CAD build for the part. Positions are in the model's coordinates, mm. A direction names the side the tool comes from. Give positions to 0.01 mm unless a question says otherwise; leave off trailing zeros. Write each loop counter-clockwise with the first axis right and the second up, starting at its lowest first coordinate (ties: lowest second). Pieces come first, ordered by that corner, then holes. Notation, with made-up numbers: (-12, -10.75) - (7, -10.75) arc R28 cw to (7, 20.25) - close; hole circle Ø8 at (-24, 46). An arc over 180 degrees is marked (long way). Answer as a JSON object with one key per item and string values.
from build123d import *

# Parameters (mm, degrees)
F0_R      = 1.778
F1_DEPTH  = 1.5875
F3_DEPTH  = 31.75
F4_R      = 2.921
F4_R_2    = 1.016
F5_DEPTH  = 7.62
F6_DEPTH  = 30.2895
F8_R      = 1.016
F9_DEPTH  = 12.7
F7_R      = 1.016
F10_DEPTH = 12.7
F11_R     = 1.016
F12_DEPTH = 12.7
F13_R     = 1.016
F14_DEPTH = 12.7


with BuildPart() as f1:
    # F0 (on Top) → F1 (new body)
    with BuildSketch(Plane.XY):
        with BuildLine():
            ThreePointArc((34.925, 0), (41.275, 6.35), (47.625, 0))
            Line((47.625, 0), (82.55, 0))
            Line((82.55, 0), (82.55, 69.85))
            Line((82.55, 69.85), (47.625, 69.85))
            ThreePointArc((47.625, 69.85), (41.275, 63.5), (34.925, 69.85))
            Line((34.925, 69.85), (0, 69.85))
            Line((0, 69.85), (0, 0))
            Line((0, 0), (34.925, 0))
        make_face()
        with BuildLine():
            Line((34.925, 69.85), (47.625, 69.85))
            ThreePointArc((47.625, 69.85), (41.275, 76.2), (34.925, 69.85))
        make_face()
        with Locations((41.275, 73.025)):
            Circle(F0_R, mode=Mode.SUBTRACT)
        with BuildLine():
            ThreePointArc((34.925, 69.85), (41.275, 63.5), (47.625, 69.85))
            Line((47.625, 69.85), (34.925, 69.85))
        make_face()
        with BuildLine():
            Line((34.925, 0), (47.625, 0))
            ThreePointArc((47.625, 0), (41.275, 6.35), (34.925, 0))
        make_face()
        with BuildLine():
            ThreePointArc((34.925, 0), (41.275, -6.35), (47.625, 0))
            Line((47.625, 0), (34.925, 0))
        make_face()
        with Locations((41.275, -3.175)):
            Circle(F0_R, mode=Mode.SUBTRACT)
    extrude(amount=F1_DEPTH)

    # F2 (on face) → F3 (join)
    with BuildSketch(Plane.XY.offset(1.5875)):
        Polygon((1.5875, 68.2625), (1.5875, 69.85), (0, 69.85), (0, 1.5875), (1.5875, 1.5875), (1.5875, 7.9375), (1.5875, 61.9125), align=None)
        Polygon((47.625, 0), (80.9625, 0), (80.9625, 1.5875), (74.6125, 1.5875), (7.9375, 1.5875), (1.5875, 1.5875), (0, 1.5875), (0, 0), (34.925, 0), align=None)
        Polygon((82.55, 0), (82.55, 69.85), (80.9625, 69.85), (80.9625, 68.2625), (80.9625, 61.9125), (80.9625, 7.9375), (80.9625, 1.5875), (80.9625, 0), align=None)
        Polygon((80.9625, 68.2625), (80.9625, 69.85), (47.625, 69.85), (34.925, 69.85), (1.5875, 69.85), (1.5875, 68.2625), (7.9375, 68.2625), (74.6125, 68.2625), align=None)
    extrude(amount=F3_DEPTH)

    # F4 (on face) → F5 (join)
    with BuildSketch(Plane.XY.offset(1.5875)):
        with Locations((10.541, 13.462)):
            Circle(F4_R)
        with Locations((10.541, 13.462)):
            Circle(F4_R_2, mode=Mode.SUBTRACT)
        with Locations((77.216, 13.462)):
            Circle(F4_R)
        with Locations((77.216, 13.462)):
            Circle(F4_R_2, mode=Mode.SUBTRACT)
        with Locations((10.541, 54.483)):
            Circle(F4_R)
        with Locations((10.541, 54.483)):
            Circle(F4_R_2, mode=Mode.SUBTRACT)
        with Locations((77.216, 54.483)):
            Circle(F4_R)
        with Locations((77.216, 54.483)):
            Circle(F4_R_2, mode=Mode.SUBTRACT)
    extrude(amount=F5_DEPTH)

    # F2 (on face) → F6 (join)
    with BuildSketch(Plane.XY.offset(1.5875)):
        with BuildLine():
            ThreePointArc((1.5875, 61.9125), (6.0776280605, 63.7723719395), (7.9375, 68.2625))
            Line((7.9375, 68.2625), (1.5875, 68.2625))
            Line((1.5875, 68.2625), (1.5875, 61.9125))
        make_face()
        with BuildLine():
            Line((80.9625, 61.9125), (80.9625, 68.2625))
            Line((80.9625, 68.2625), (74.6125, 68.2625))
            ThreePointArc((74.6125, 68.2625), (76.4723719395, 63.7723719395), (80.9625, 61.9125))
        make_face()
        with BuildLine():
            Line((1.5875, 1.5875), (7.9375, 1.5875))
            ThreePointArc((7.9375, 1.5875), (6.0776280605, 6.0776280605), (1.5875, 7.9375))
            Line((1.5875, 7.9375), (1.5875, 1.5875))
        make_face()
        with BuildLine():
            Line((74.6125, 1.5875), (80.9625, 1.5875))
            Line((80.9625, 1.5875), (80.9625, 7.9375))
            ThreePointArc((80.9625, 7.9375), (76.4723719395, 6.0776280605), (74.6125, 1.5875))
        make_face()
    extrude(amount=F6_DEPTH)

    # F8 (on face) → F9 (cut)
    with BuildSketch(Plane.XY.offset(31.877)):
        with Locations((78.7174359697, 3.8325640303)):
            Circle(F8_R)
    extrude(amount=-F9_DEPTH, mode=Mode.SUBTRACT)

    # F7 (on face) → F10 (cut)
    with BuildSketch(Plane.XY.offset(31.877)):
        with Locations((3.8325640303, 3.8325640303)):
            Circle(F7_R)
    extrude(amount=-F10_DEPTH, mode=Mode.SUBTRACT)

    # F11 (on face) → F12 (cut)
    with BuildSketch(Plane.XY.offset(31.877)):
        with Locations((3.8325640303, 66.0174359697)):
            Circle(F11_R)
    extrude(amount=-F12_DEPTH, mode=Mode.SUBTRACT)

    # F13 (on face) → F14 (cut)
    with BuildSketch(Plane.XY.offset(31.877)):
        with Locations((78.7174359697, 66.0174359697)):
            Circle(F13_R)
    extrude(amount=-F14_DEPTH, mode=Mode.SUBTRACT)


solid = f1.part
Item 1: Which spindle directions (+Z, -Z, +X, -X, +Y, -Y) get a long thin tool onto all of the face, cutting with end or side? Do faces 4 (the flat face through (41, 36, 0)), 5 (the flat face through (78, 65, 31.877)). Say none if no direction does.
Entries:
{"face 4": "-Z, +X, -X, +Y, -Y", "face 5": "+Z"}
Item 2: Cut at C-C (x = 38). Give the cut face in (y, z).
Entries:
{"outline": "(-5.44, 0) - (75.29, 0) - (75.29, 1.59) - (69.85, 1.59) - (69.85, 33.34) - (68.26, 33.34) - (68.26, 1.59) - (1.59, 1.59) - (1.59, 33.34) - (0, 33.34) - (0, 1.59) - (-5.44, 1.59) - close"}
Item 3: Mould opens along Y. For faces 1 (the cylindrical face through (41.14, -6.35, 0.78)), 2 (the flat face through (12, 14, 9.208)), 3 (the flat face through (0, 35, 16)) say: +Y half, -Y half, draft (parallel to the pull), parting line (faces both ways), or undercut.
Entries:
{"face 1": "-Y half", "face 2": "undercut", "face 3": "draft"}
Item 4: Flat gauge pins, fed straight in: P1, Ø0.6, axis at x = 79, y = 3.5, coming from the +Z side; P2, Ø5, axis at x = 9, y = 26, coming from the +Z side; P3, Ø1.9, axis at x = 4.5, y = 65.5, coming from the +Z side. Where does each tip first touch, or does it go through?
Entries:
{"P1": "z = 19.18", "P2": "z = 1.59", "P3": "z = 31.88"}
Item 5: Probe line 1 (X direction, y = 54.5, z = 28); line 2 (Y direction, x = 19.5, z = 23.5); line 3 (X direction, y = 2, z = 20.5). List the from-to ranges inside material, lowest first. Write a range as from..to.
Entries:
{"line 1": "0..1.59, 80.96..82.55", "line 2": "0..1.59, 68.26..69.85", "line 3": "0..7.92, 74.63..82.55"}
Item 6: Cut at B-B (z = 4.5). State how many separate pieces and enclosed holes the cut face has, and give its area (3 significant figures).
Entries:
{"separate pieces": "5", "enclosed holes": "5", "area": "695 mm2"}
Item 7: Cut at A-A (y = 40.5). Give the cut face in (x, z).
Entries:
{"outline": "(0, 0) - (82.55, 0) - (82.55, 33.34) - (80.96, 33.34) - (80.96, 1.59) - (1.59, 1.59) - (1.59, 33.34) - (0, 33.34) - close"}
